from build123d import *

# Parameters (mm, degrees)
SKETCH1_R           = 167.5
SKETCH1_R_2         = 4
SKETCH1_R_3         = 90
BOSS_EXTRUDE1_DEPTH = 6
SKETCH4_OUTSIDE_W   = 431.76
SKETCH4_OUTSIDE_H   = 431.76
SKETCH4_OUTSIDE_W_2 = 330
SKETCH4_OUTSIDE_H_2 = 330
CUT_EXTRUDE3_DEPTH  = 10


with BuildPart() as part:
    # Sketch1 → Boss-Extrude1 (new body)
    with BuildSketch(Plane(origin=(0, 0, 0), x_dir=(1, 0, 0), z_dir=(0, 1, 0))):
        with Locations(Location((0, 0, 0), (0, 0, 270))):
            Circle(SKETCH1_R)
        with Locations(Location((0, 115, 0), (0, 0, 270))):
            Circle(SKETCH1_R_2, mode=Mode.SUBTRACT)
        with Locations(Location((0, 0, 0), (0, 0, 270))):
            Circle(SKETCH1_R_3, mode=Mode.SUBTRACT)
        with Locations(Location((-137, 0, 0), (0, 0, 270))):
            Circle(SKETCH1_R_2, mode=Mode.SUBTRACT)
        with Locations(Location((-158, 0, 0), (0, 0, 270))):
            Circle(SKETCH1_R_2, mode=Mode.SUBTRACT)
        with Locations(Location((0, -158, 0), (0, 0, 270))):
            Circle(SKETCH1_R_2, mode=Mode.SUBTRACT)
        with Locations(Location((0, -137, 0), (0, 0, 270))):
            Circle(SKETCH1_R_2, mode=Mode.SUBTRACT)
        with Locations(Location((81.317279836, 81.317279836, 0), (0, 0, 270))):
            Circle(SKETCH1_R_2, mode=Mode.SUBTRACT)
        with Locations(Location((115, 0, 0), (0, 0, 270))):
            Circle(SKETCH1_R_2, mode=Mode.SUBTRACT)
        with Locations(Location((81.317279836, -81.317279836, 0), (0, 0, 270))):
            Circle(SKETCH1_R_2, mode=Mode.SUBTRACT)
        with Locations(Location((0, -115, 0), (0, 0, 270))):
            Circle(SKETCH1_R_2, mode=Mode.SUBTRACT)
        with Locations(Location((-81.317279836, -81.317279836, 0), (0, 0, 270))):
            Circle(SKETCH1_R_2, mode=Mode.SUBTRACT)
        with Locations(Location((-115, 0, 0), (0, 0, 270))):
            Circle(SKETCH1_R_2, mode=Mode.SUBTRACT)
        with Locations(Location((-81.317279836, 81.317279836, 0), (0, 0, 270))):
            Circle(SKETCH1_R_2, mode=Mode.SUBTRACT)
        with Locations(Location((0, 137, 0), (0, 0, 270))):
            Circle(SKETCH1_R_2, mode=Mode.SUBTRACT)
        with Locations(Location((0, 158, 0), (0, 0, 270))):
            Circle(SKETCH1_R_2, mode=Mode.SUBTRACT)
        with Locations(Location((137, 0, 0), (0, 0, 270))):
            Circle(SKETCH1_R_2, mode=Mode.SUBTRACT)
        with Locations(Location((158, 0, 0), (0, 0, 270))):
            Circle(SKETCH1_R_2, mode=Mode.SUBTRACT)
    extrude(amount=BOSS_EXTRUDE1_DEPTH)

    # Sketch4 outside → Cut-Extrude3 (cut)
    with BuildSketch(Plane(origin=(0, 6, 0), x_dir=(1, 0, 0), z_dir=(0, 1, 0))):
        Rectangle(SKETCH4_OUTSIDE_W, SKETCH4_OUTSIDE_H)
        Rectangle(SKETCH4_OUTSIDE_W_2, SKETCH4_OUTSIDE_H_2, mode=Mode.SUBTRACT)
    extrude(amount=-CUT_EXTRUDE3_DEPTH, mode=Mode.SUBTRACT)


solid = part.part
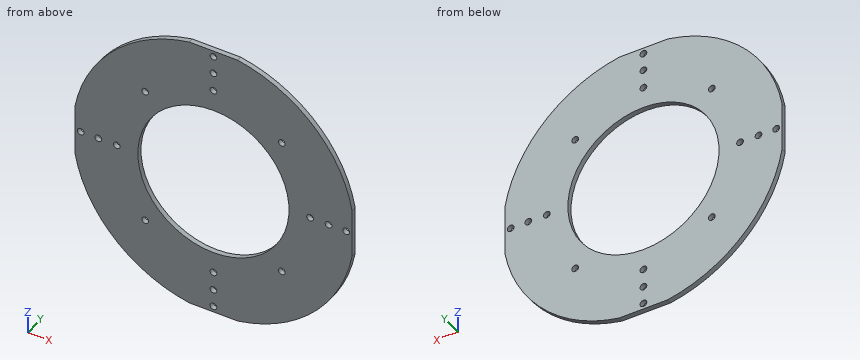
CAD build for the part. Positions are in the model's coordinates, mm. Round coordinates to 2 decimals unless told otherwise and drop trailing zeros. Order: outer loops, then holes, each group sorted by start corner. A loop starts at its lowest first (then second) coordinate and runs counter-clockwise, first axis right, second up. Notation, with made-up numbers: (-26.5, -26) - (17.5, -26) arc R24 ccw to (17.5, 6) - close; hole circle Ø3 at (-16.75, 10). An arc over 180 degrees is marked (long way). Return JSON: item names as keys, results as strings.
(1) Pin check, flat tips, straight feed: pin 1 Ø10.5 at (x, z) = (-81.32, -81.32) entering from -Y; pin 2 Ø5 at (x, z) = (0, -137) entering from -Y; pin 3 Ø1 at (y, z) = (2, 61.5) entering from +X; pin 4 Ø3 at (x, y) = (-63.5, 2) entering from +Z. Stop position of each tip, or through.
Answer key:
{"pin 1": "stops at y = 0", "pin 2": "passes through", "pin 3": "stops at x = 156", "pin 4": "stops at z = 155.6"}
(2) Wall check: probe 1 along X at (y, z) = (2.9, -115); probe 2 along Z at (x, y) = (113, 5.15); probe 3 along Z at (x, y) = (-74.5, 0.2). Give the ranges that are in metal, low to high. Write a range as from..to.
Answer key:
{"probe 1": "x = -121.78..-4, 4..121.78", "probe 2": "z = -123.64..-3.46, 3.46..123.64", "probe 3": "z = -150.02..-50.5, 50.5..150.02"}
(3) Cut at A-A (z = 50). Give the cut face in (x, y), then the cut area to 3 significant figures.
Answer key:
{"outline": "(-159.86, 0) - (-74.83, 0) - (-74.83, 6) - (-159.86, 6) - close; (74.83, 0) - (159.86, 0) - (159.86, 6) - (74.83, 6) - close", "area": "1,020 mm^2"}
(4) Cut at B-B (x = -115). Give the cut face in (y, z).
Answer key:
{"outline": "(0, -121.78) - (6, -121.78) - (6, -4) - (0, -4) - close; (0, 4) - (6, 4) - (6, 121.78) - (0, 121.78) - close"}
(5) Cut at C-C (y = 4). State how many separate pieces and enclosed holes the cut face has, then the cut area to 3 significant figures.
Answer key:
{"separate pieces": "1", "enclosed holes": "17", "area": "61,500 mm^2"}
